Source: CAD feature listing. Evaluate the final solid. Frame: model axes, mm. Face numbers are marked on the shaded views. A direction names the side the tool comes from. Give positions to 0.01 mm unless a question says otherwise; leave off trailing zeros. Order: outer loops, then holes, each group sorted by start corner. A loop starts at its lowest first (then second) coordinate and runs counter-clockwise, first axis right, second up. Notation, with made-up numbers: (1.5, 55.5) -> (15.5, 55.5) arc R12 ccw to (15.5, 77.5) -> close; hole circle Ø1 at (-4.75, 17.25). An arc over 180 degrees is marked (long way). Answer in a Markdown table with one row per item.
```python
from build123d import *

# Parameters (mm, degrees)
CYLINDER_R          = 3.5
CYLINDER_DEPTH      = 5
CYLINDER_ROLL_ANGLE = 90
PAD_DEPTH           = 10
FILLET_R            = 1.437
SKETCH001_R         = 2.2
POCKET_DEPTH        = 5
FILLET001_R         = 1


with BuildPart() as cylinder:
    # Cylinder → Cylinder (new body)
    with BuildSketch(Plane.XY):
        Circle(CYLINDER_R)
    extrude(amount=CYLINDER_DEPTH)


with BuildPart() as cylinder_1:
    # Cylinder roll: moved
    add(cylinder.part.rotate(Axis((0, 0, 0), (1, 0, 0)), CYLINDER_ROLL_ANGLE))


with BuildPart() as cylinder_2:
    # Cylinder placement: moved
    add(cylinder_1.part.moved(Location((0, 9, 5))))


with BuildPart() as fillet001:
    # Sketch → Pad (new body)
    with BuildSketch(Plane.XY):
        with BuildLine():
            ThreePointArc((4, -3.774917), (0, 5.5), (-4, -3.774917))
            Line((-4, -3.774917), (-4.5, -6))
            ThreePointArc((-6.344289, 4), (-7.375612, -1.360276), (-4.5, -6))
            Line((-6.344289, 4), (-10, 4))
            Line((-10, 4), (-10, 10))
            Line((-10, 10), (10, 10))
            Line((10, 10), (10, 4))
            Line((10, 4), (6.344289, 4))
            ThreePointArc((4.5, -6), (7.375612, -1.360276), (6.344289, 4))
            Line((4, -3.774917), (4.5, -6))
        make_face()
    extrude(amount=PAD_DEPTH)

    # Fillet
    fillet_edges = [fillet001.edges().sort_by_distance(p)[0] for p in [
        (-6.344289, 4, 5),
        (-10, 4, 5),
        (10, 4, 5),
        (6.344289, 4, 5),
    ]]
    fillet(fillet_edges, radius=FILLET_R)

    # Sketch001 → Pocket (cut)
    with BuildSketch(Plane(origin=(0, 10, 0), x_dir=(-1, 0, 0), z_dir=(0, 1, 0))):
        with Locations((0, 5)):
            Circle(SKETCH001_R)
    extrude(amount=-POCKET_DEPTH, mode=Mode.SUBTRACT)

    # Cut: cut Cylinder
    add(cylinder_2.part, mode=Mode.SUBTRACT)

    # Fillet001
    fillet001_edges = [fillet001.edges().sort_by_distance(p)[0] for p in [
        (10, 7.7185, 10),
        (10, 7.7185, 0),
        (-10, 7.7185, 0),
        (-10, 7.7185, 10),
    ]]
    fillet(fillet001_edges, radius=FILLET001_R)


solid = fillet001.part
```
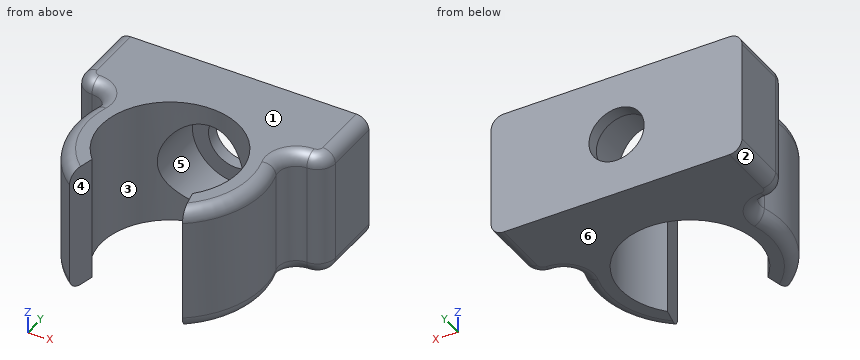
(1) Access query for the marked faces 4, 5 and 6. Directions: +Z, -Z, +X, -X, +Y, -Y. A direction counts if a zero-diameter tool reaches every point of the face in a straight line with its end or side. Return the directions, or none.
A:
| item | result |
|---|---|
| face 4 | +Z, -Z, -Y |
| face 5 | -Y |
| face 6 | -Z, +X, -X, +Y, -Y |
(2) Section query C-C (x = -3.75). Return the cut outline in (y, z).
A:
| item | result |
|---|---|
| outline | (4.02, 0) -> (10, 0) -> (10, 10) -> (4.02, 10) -> close |
(3) Section query A-A (x = 0). Return the cut outline in (y, z).
A:
| item | result |
|---|---|
| outline | (5.5, 0) -> (10, 0) -> (10, 2.8) -> (9, 2.8) -> (9, 1.5) -> (5.5, 1.5) -> close; (5.5, 8.5) -> (9, 8.5) -> (9, 7.2) -> (10, 7.2) -> (10, 10) -> (5.5, 10) -> close |
(4) Pull-direction query (X, two-part tool) for the marked faces 1, 2 and 3; classes: +X half, -X half, draft (parallel to the pull), parting line (faces both ways), or undercut.
A:
| item | result |
|---|---|
| face 1 | draft |
| face 2 | -X half |
| face 3 | undercut |
(5) Ray query, probe 1 along Z at (x, y) = (0, 9.65); probe 2 along X at (y, z) = (0, 3.5); probe 3 along X at (y, z) = (6.8, 5). Return the intervals inside material, ascending.
A:
| item | result |
|---|---|
| probe 1 | z = 0 to 2.8, 7.2 to 10 |
| probe 2 | x = -7.5 to -5.5, 5.5 to 7.5 |
| probe 3 | x = -10 to -3.5, 3.5 to 10 |
